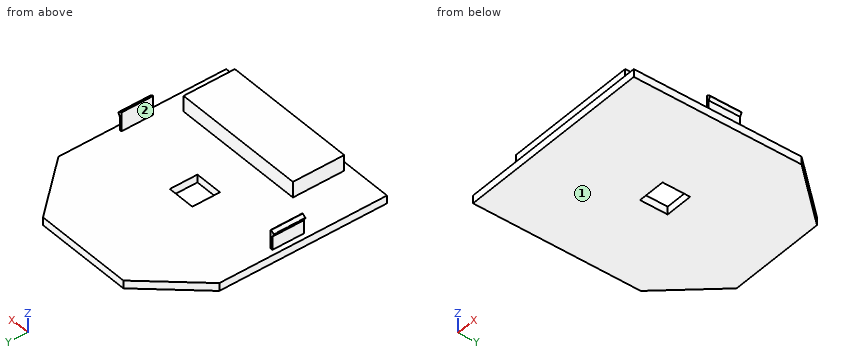
```python
from build123d import *

# Parameters (mm, degrees)
BOSS_EXTRU_1_DEPTH      = 4
ESQUISSE4_W             = 68
ESQUISSE4_H             = 26
BOSS_EXTRU_3_DEPTH      = 8
ESQUISSE8_W             = 14
ESQUISSE8_H             = 14
ENL_V_MAT_EXTRU_2_DEPTH = 13
ESQUISSE10_W            = 1
ESQUISSE10_H            = 16
BOSS_EXTRU_4_DEPTH      = 8.5
BOSS_EXTRU_5_DEPTH      = 16
BOSS_EXTRU_6_DEPTH      = 16
CONG_1_R                = 0.25
CONG_2_R                = 0.25


with BuildPart() as part:
    # Esquisse1 → Boss.-Extru.1 (new body)
    with BuildSketch(Plane.XY):
        Polygon((0, 0), (0, 85), (25, 113.20056997), (75, 113.20056997), (100, 85), (100, 0), align=None)
    extrude(amount=BOSS_EXTRU_1_DEPTH)

    # Esquisse4 → Boss.-Extru.3 (add)
    with BuildSketch(Plane.XY.offset(4)):
        with Locations((56.41, 16.41)):
            Rectangle(ESQUISSE4_W, ESQUISSE4_H)
    extrude(amount=BOSS_EXTRU_3_DEPTH)

    # Esquisse8 → Enlèv. mat.-Extru.2 (cut, through all)
    with BuildSketch(Plane(origin=(0, 0, 0), x_dir=(-1, 0, 0), z_dir=(0, 0, -1))):
        with Locations((-50, 56.60056997)):
            Rectangle(ESQUISSE8_W, ESQUISSE8_H)
    extrude(amount=-ENL_V_MAT_EXTRU_2_DEPTH, mode=Mode.SUBTRACT)

    # Esquisse10 → Boss.-Extru.4 (add)
    with BuildSketch(Plane.XY.offset(4)):
        with Locations((3.1, 48)):
            Rectangle(ESQUISSE10_W, ESQUISSE10_H)
        with Locations((96.9, 48)):
            Rectangle(ESQUISSE10_W, ESQUISSE10_H)
    extrude(amount=BOSS_EXTRU_4_DEPTH)

    # Esquisse13 → Boss.-Extru.5 (add)
    with BuildSketch(Plane(origin=(0, 40, 0), x_dir=(-1, 0, 0), z_dir=(0, -1, 0))):
        Polygon((-98.4, -12.5), (-97.4, -10.767949192), (-97.4, -12.5), (-96.4, -12.5), (-96.4, -14), align=None)
    extrude(amount=-BOSS_EXTRU_5_DEPTH)

    # Esquisse14 → Boss.-Extru.6 (add)
    with BuildSketch(Plane.XZ.offset(-40)):
        Polygon((1.6, 12.5), (2.6, 10.767949192), (2.6, 12.5), (3.6, 12.5), (3.6, 14), align=None)
    extrude(amount=-BOSS_EXTRU_6_DEPTH)

    # Congé1
    cong_1_edges = [part.edges().sort_by_distance(p)[0] for p in [
        (98.4, 48, 12.5),
        (1.6, 48, 12.5),
    ]]
    fillet(cong_1_edges, radius=CONG_1_R)

    # Congé2
    cong_2_edges = [part.edges().sort_by_distance(p)[0] for p in [
        (96.4, 48, 14),
        (3.6, 48, 14),
    ]]
    fillet(cong_2_edges, radius=CONG_2_R)


solid = part.part
```
Verification items for the finished model (mm, model axes). Face numbers are marked on the shaded views. Coordinates: 2 decimals unless noted, no trailing zeros. Order: outer loops, then holes, each group sorted by start corner. A loop starts at its lowest first (then second) coordinate and runs counter-clockwise, first axis right, second up. Notation, with made-up numbers: (20, 72) -> (54, 72) arc R17 ccw to (54, 85) -> close; hole circle Ø6 at (30, 6.5). An arc over 180 degrees is marked (long way). Put each result on its own line as item: value. Start each with the question number.
1) Release check for a two-part mould opening along X. For the marked faces 1 and 2 record: pulls with the +X half, pulls with the -X half, needs draft (parallel to the pull), parting line crosses it, or undercut.
2) Cross-section at D-D (z = 2.75). Enter the section's corners in (x, y).
3) Go/stop test with flat-tipped pins: pin 1 (3 mm diameter, centred on y = 44, z = 6.5, fed in from +X); pin 2 (8 mm diameter, centred on x = 75.5, z = 9, fed in from +Y); pin 3 (1.5 mm diameter, centred on x = 2.5, z = 8, fed in from -Y). Record where each tip stops, or that it passes through.
4) Cross-section at C-C (x = 34). Enter the section's corners in (y, z).
5) Cross-section at B-B (y = 53.5). Enter the section's corners in (x, z), plus the area to 3 significant figures.
6) Material ranges on L1, parallel to Y at x = 44.5, z = 1.25; L2, parallel to Z at x = 48, y = 75.5; L3, parallel to Y at x = 60.5, z = 8.5, recorded low to high.
7) Cross-section at A-A (z = 9.5). Enter the section's corners in (x, y).
Geometry check:
1. face 1: needs draft
1. face 2: undercut
2. outline: (0, 0) -> (100, 0) -> (100, 85) -> (75, 113.2) -> (25, 113.2) -> (0, 85) -> close; hole (43, 49.6) -> (57, 49.6) -> (57, 63.6) -> (43, 63.6) -> close
3. pin 1: stops at x = 97.4
3. pin 2: stops at y = 29.41
3. pin 3: stops at y = 40
4. outline: (0, 0) -> (113.2, 0) -> (113.2, 4) -> (29.41, 4) -> (29.41, 12) -> (3.41, 12) -> (3.41, 4) -> (0, 4) -> close
5. outline: (0, 0) -> (43, 0) -> (43, 4) -> (3.6, 4) -> (3.6, 13.5) arc R0.25 ccw to (3.2, 13.7) -> (1.78, 12.63) arc R0.25 ccw to (1.71, 12.31) -> (2.6, 10.77) -> (2.6, 4) -> (0, 4) -> close; (57, 0) -> (100, 0) -> (100, 4) -> (97.4, 4) -> (97.4, 10.77) -> (98.29, 12.31) arc R0.25 ccw to (98.22, 12.63) -> (96.8, 13.7) arc R0.25 ccw to (96.4, 13.5) -> (96.4, 4) -> (57, 4) -> close
5. area: 366 mm^2
6. L1: y = 0 to 49.6, 63.6 to 113.2
6. L2: z = 0 to 4
6. L3: y = 3.41 to 29.41
7. outline: (2.6, 40) -> (3.6, 40) -> (3.6, 56) -> (2.6, 56) -> close; (22.41, 3.41) -> (90.41, 3.41) -> (90.41, 29.41) -> (22.41, 29.41) -> close; (96.4, 40) -> (97.4, 40) -> (97.4, 56) -> (96.4, 56) -> close
